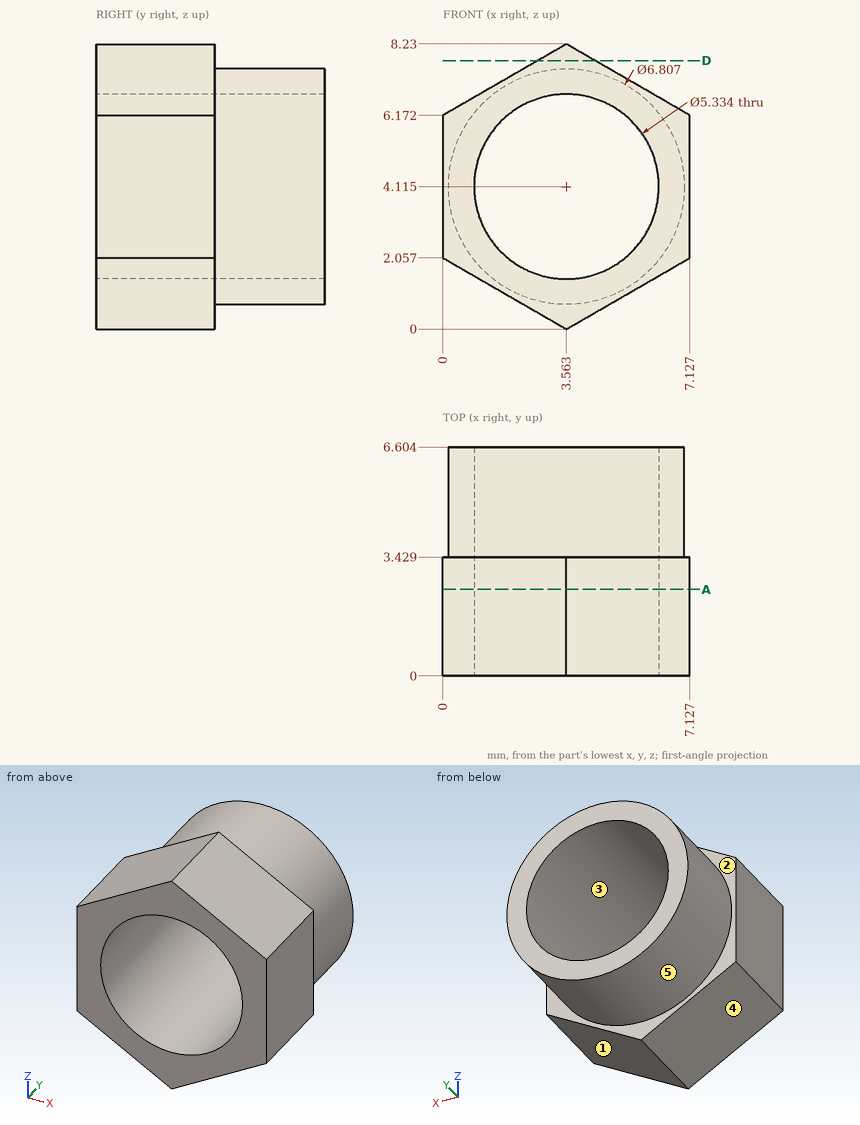
Can you work these out from the drawing? Everything is in mm from the part's minimum corner. A direction names the side the tool comes from. Give positions to 0.01 mm unless a question says otherwise; leave off trailing zeros. Order: outer loops, then holes, each group sorted by start corner. A loop starts at its lowest first (then second) coordinate and runs counter-clockwise, first axis right, second up. Notation, with made-up numbers: M 20.5,87.5 L 37.5,87.5 A11 ccw 37.5,103.5 Z; hole C 84,-27 d4. An arc over 180 degrees is marked long. One line per item, written item: value.
Item 1: If we mould it in two halves opening along Z, with no side actions, what happens to the marked faces 3, 4 and 5? For each: pulls with the +Z half, pulls with the -Z half, needs draft (parallel to the pull), parting line crosses it, or undercut.
Verdict:
face 3: undercut
face 4: pulls with the -Z half
face 5: parting line crosses it
Item 2: For the marked faces 1 and 2, which set-ups out of +Z, -Z, +X, -X, +Y, -Y let a thin tool reach every point of the face, with its end or its side?
Verdict:
face 1: -Z, +X, +Y, -Y
face 2: +Y
Item 3: Please list where these lines run through material, in increasing order: line 1 (X direction, y = 3.25, z = 2) (1 decimal); line 2 (Z direction, x = 1.5, y = 2) (1 decimal); line 3 (Z direction, x = 3, y = 2.75) (1 decimal).
Verdict:
line 1: 0.1 to 1.9, 5.2 to 7
line 2: 1.2 to 2.4, 5.8 to 7
line 3: 0.3 to 1.5, 6.7 to 7.9
Item 4: If we section it at A-A on y = 2.5: Write out the boundary of the cut face in (x, z) (1 decimal).
Verdict:
outline: M 0,2.1 L 3.6,0 L 7.1,2.1 L 7.1,6.2 L 3.6,8.2 L 0,6.2 Z; hole C 3.6,4.1 d5.3
Item 5: For pin 1 (1.5 mm diameter, centred on y = 4.5, z = 5.5, fed in from -X), with a flat end and sliding along its axis, tell me the tip position at first contact or that it passes through.
Verdict:
pin 1: x = 0.22
Item 6: If we section it at D-D on z = 7.75: Write out the boundary of the cut face in (x, y) (1 decimal).
Verdict:
outline: M 2.7,0 L 4.4,0 L 4.4,3.4 L 2.7,3.4 Z
